Read the model definition and answer for the solid it produces. Units are mm, in the model's axes. Face numbers are marked on the shaded views. Coordinates: 2 decimals unless noted, no trailing zeros. Loops run counter-clockwise (first coordinate to the right, second up) from the corner with the lowest first, then second, coordinate; pieces in that order, holes last. Notation, with made-up numbers: (43, 3) - (80, 3) arc R7 ccw to (80, 8) - close; hole circle Ø8 at (61.25, 83). An arc over 180 degrees is marked (long way). Use one line per item in the form item = value. Start each with the question number.
1) A cutting plane is placed at B-B (x = 0). Give the vertices of the cut face in (y, z), and give its area (3 significant figures).
2) A cutting plane is placed at C-C (y = 0.45). Give the vertices of the cut face in (x, z), and give its area (3 significant figures).
3) The mould has two halves that part along Z. Classify the marked faces 1, 2 and 3: released by +Z, released by -Z, zero draft, split by the parting line, or undercut.
4) A cutting plane is placed at D-D (z = 8). Give the vertices of the cut face in (x, y), and give its area (3 significant figures).
5) Each of these flat-tipped pins is pushed along its axis until it touches: P1, Ø2, axis at x = -4.5, z = -3.5, coming from the +Y side; P2, Ø2, axis at x = 8, z = 0, coming from the -Y side; P3, Ø1, axis at x = -2.5, y = 3, coming from the -Z side. Where does it stop, or does it pass through?
6) A cutting plane is placed at A-A (z = 0). Give the vertices of the cut face in (x, y).
7) Consider line 1 (Z direction, x = 0, y = 1.45); line 2 (Z direction, x = 0, y = 2.2). Determine where each line is inside the solid, lowest interval first.
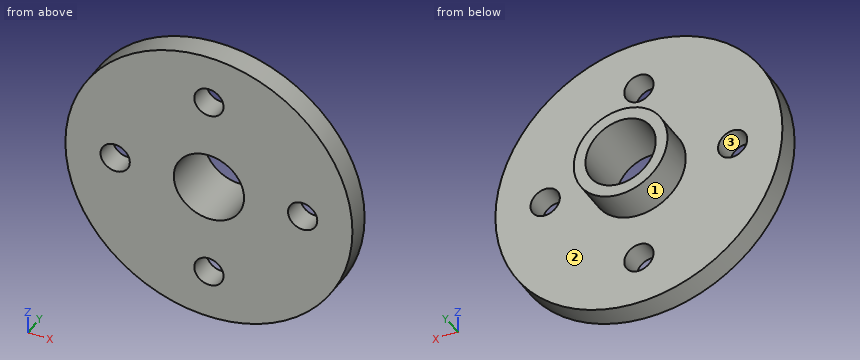
from build123d import *

# Parameters (mm, degrees)
SKETCH_1_R      = 12.25
SKETCH_1_R_2    = 3
SKETCH_1_R_3    = 1.25
EXTRUDE_1_DEPTH = 2
SKETCH_2_R      = 4
SKETCH_2_R_2    = 3
EXTRUDE_2_DEPTH = 3


with BuildPart() as part:
    # 草图1 → 凸台-拉伸1 (new body)
    with BuildSketch(Plane(origin=(0, 0, 0), x_dir=(1, 0, 0), z_dir=(0, 1, 0))):
        Circle(SKETCH_1_R)
        Circle(SKETCH_1_R_2, mode=Mode.SUBTRACT)
        with Locations((8, 0)):
            Circle(SKETCH_1_R_3, mode=Mode.SUBTRACT)
        with Locations((0, -8)):
            Circle(SKETCH_1_R_3, mode=Mode.SUBTRACT)
        with Locations((-8, 0)):
            Circle(SKETCH_1_R_3, mode=Mode.SUBTRACT)
        with Locations((0, 8)):
            Circle(SKETCH_1_R_3, mode=Mode.SUBTRACT)
    extrude(amount=EXTRUDE_1_DEPTH)

    # 草图2 → 凸台-拉伸2 (add)
    with BuildSketch(Plane(origin=(0, 2, 0), x_dir=(1, 0, 0), z_dir=(0, 1, 0))):
        Circle(SKETCH_2_R)
        Circle(SKETCH_2_R_2, mode=Mode.SUBTRACT)
    extrude(amount=EXTRUDE_2_DEPTH)


solid = part.part
Found:
q1.outline = (0, -12.25) - (2, -12.25) - (2, -9.25) - (0, -9.25) - close; (0, -6.75) - (2, -6.75) - (2, -4) - (5, -4) - (5, -3) - (0, -3) - close; (0, 3) - (5, 3) - (5, 4) - (2, 4) - (2, 6.75) - (0, 6.75) - close; (0, 9.25) - (2, 9.25) - (2, 12.25) - (0, 12.25) - close
q1.area = 33.0 mm^2
q2.outline = circle Ø24.5 at (0, 0); hole circle Ø2.5 at (-8, 0); hole circle Ø6 at (0, 0); hole circle Ø2.5 at (0, -8); hole circle Ø2.5 at (0, 8); hole circle Ø2.5 at (8, 0)
q2.area = 424 mm^2
q3.face_1 = split by the parting line
q3.face_2 = zero draft
q3.face_3 = undercut
q4.outline = (-9.28, 0) - (-1.25, 0) - (-1.25, 2) - (-9.28, 2) - close; (1.25, 0) - (9.28, 0) - (9.28, 2) - (1.25, 2) - close
q4.area = 32.1 mm^2
q5.P1 = 2
q5.P2 = through
q5.P3 = -3.46
q6.outline = (-12.25, 0) - (-9.25, 0) - (-9.25, 2) - (-12.25, 2) - close; (-6.75, 0) - (-3, 0) - (-3, 5) - (-4, 5) - (-4, 2) - (-6.75, 2) - close; (3, 0) - (6.75, 0) - (6.75, 2) - (4, 2) - (4, 5) - (3, 5) - close; (9.25, 0) - (12.25, 0) - (12.25, 2) - (9.25, 2) - close
q7.line_1 = -12.25 to -9.25, -6.75 to -3, 3 to 6.75, 9.25 to 12.25
q7.line_2 = -4 to -3, 3 to 4
